from build123d import *

# Parameters (mm, degrees)
SKETCH_R     = 7.5
PAD_DEPTH    = 7
CHAMFER_SIZE = 0.6


with BuildPart() as part:
    # Sketch → Pad (new body)
    with BuildSketch(Plane.XY):
        Circle(SKETCH_R)
        with BuildLine():
            ThreePointArc((-2.5, 3.122499), (-3.518971, 1.901799), (-3.981855, 0.380567))
            Line((-5.478695, -0.483634), (-3.981855, 0.380567))
            ThreePointArc((-5.478695, -0.483634), (-4.659167, -2.922699), (-2.81991, -4.722087))
            Line((-1.232265, -3.80546), (-2.81991, -4.722087))
            ThreePointArc((-1.232265, -3.80546), (0.117848, -3.998264), (1.454262, -3.726275))
            Line((2.992718, -4.614503), (1.454262, -3.726275))
            ThreePointArc((2.992718, -4.614503), (4.763149, -2.749985), (5.492638, -0.284484))
            Line((3.954108, 0.604177), (5.492638, -0.284484))
            ThreePointArc((3.954108, 0.604177), (3.46401, 2.000159), (2.5, 3.122499))
            Line((2.5, 3.122499), (2.5, 4.898979))
            ThreePointArc((2.5, 4.898979), (0, 5.5), (-2.5, 4.898979))
            Line((-2.5, 3.122499), (-2.5, 4.898979))
        make_face(mode=Mode.SUBTRACT)
    extrude(amount=PAD_DEPTH)

    # Chamfer
    chamfer_edges = [part.edges().sort_by_distance(p)[0] for p in [
        (-3.518971, 1.901799, 7),
        (-4.730275, -0.051534, 7),
        (-4.659167, -2.922699, 7),
        (-2.026088, -4.263773, 7),
        (0.117848, -3.998264, 7),
        (2.22349, -4.170389, 7),
        (4.763149, -2.749985, 7),
        (4.723373, 0.159847, 7),
        (3.46401, 2.000159, 7),
        (2.5, 4.010739, 7),
        (0, 5.5, 7),
        (-2.5, 4.010739, 7),
    ]]
    chamfer(chamfer_edges, length=CHAMFER_SIZE)


solid = part.part
CAD build for the part. Positions are in the model's coordinates, mm. A direction names the side the tool comes from. Round coordinates to 2 decimals unless told otherwise and drop trailing zeros. Loops run counter-clockwise (first coordinate to the right, second up) from the corner with the lowest first, then second, coordinate; pieces in that order, holes last.
(1) Cut at C-C (y = 4). Give the cut face in (x, z), plus the area to 3 significant figures.
(2) Cut at B-B (z = 5). Give the cut face in (x, y).
(3) Drop flat-ended pins along their axis: pin 1 (0.9 mm diameter, centred on y = 4, z = 2, fed in from +X); pin 2 (0.5 mm diameter, centred on y = 4, z = 3, fed in from -X); pin 3 (1.5 mm diameter, centred on x = -2, z = 3, fed in from -Y). Give the stop position or say it passes through.
(4) Cut at D-D (x = -6.5). Give the cut face in (y, z), plus the area to 3 significant figures.
(5) Which spindle directions (+Z, -Z, +X, -X, +Y, -Y) get a long thin tool onto all of the face, cutting with end or side? Do faces 1 (the conical face through (0.1, -4.2, 6.6)), 2 (the flat face through (5, 2, 7)), 3 (the flat face through (-2.015, -4.257, 3.155)). Say none if no direction does.
(6) Wall check: line 1 along X through (y, z) = (-1, 2.25); line 2 along X through (y, z) = (5, 3); line 3 along Y through (x, z) = (3.25, 2). Give the ranges that are in metal, low to high.
(7) Cut at A-A (x = 0). Give the cut face in (y, z), plus the area to 3 significant figures.
(8) Two-plate mould, pull along Y, no slides. Class faces 4 (the conical face through (3.681, 2.1, 6.638)), 5 (the flat face through (0, -5, 0)), 6 (the cylindrical face through (-7.493, 0.33, 3.451)): +Y half, -Y half, draft (parallel to the pull), parting line (faces both ways), or undercut.
Findings below:
1. outline: (-6.34, 0) - (-2.5, 0) - (-2.5, 6.4) - (-3.1, 7) - (-6.34, 7) - close; (2.5, 0) - (6.34, 0) - (6.34, 7) - (3.1, 7) - (2.5, 6.4) - close
1. area: 53.5 mm2
2. outline: circle Ø15 at (0, 0); hole (-5.48, -0.48) arc R5.5 ccw to (-2.82, -4.72) - (-1.23, -3.81) arc R4 ccw to (1.45, -3.73) - (2.99, -4.61) arc R5.5 ccw to (5.49, -0.28) - (3.95, 0.6) arc R4 ccw to (2.5, 3.12) - (2.5, 4.9) arc R5.5 ccw to (-2.5, 4.9) - (-2.5, 3.12) arc R4 ccw to (-3.98, 0.38) - close
3. pin 1: stops at x = 6.61
3. pin 2: stops at x = -6.5
3. pin 3: stops at y = -7.4
4. outline: (-3.74, 0) - (3.74, 0) - (3.74, 7) - (-3.74, 7) - close
4. area: 52.4 mm2
5. face 1: +Z
5. face 2: +Z, +X, -X, +Y, -Y
5. face 3: +Z, -Z
6. line 1: x = -7.43 to -5.41, 5.41 to 7.43
6. line 2: x = -5.59 to -2.29, 2.29 to 5.59
6. line 3: y = -6.76 to -4.44, 2.33 to 6.76
7. outline: (-7.5, 0) - (-4, 0) - (-4, 6.4) - (-4.6, 7) - (-7.5, 7) - close; (5.5, 0) - (7.5, 0) - (7.5, 7) - (6.1, 7) - (5.5, 6.4) - close
7. area: 38.1 mm2
8. face 4: undercut
8. face 5: draft
8. face 6: parting line
